The listing builds one solid part. Answer for the finished solid, in the listing's coordinates (mm). Round coordinates to 2 decimals unless told otherwise and drop trailing zeros. Loops run counter-clockwise (first coordinate to the right, second up) from the corner with the lowest first, then second, coordinate; pieces in that order, holes last. Notation, with made-up numbers: M -39.75,-36.5 L -27.75,-36.5 A13 cw -27.75,-20.5 Z; hole C 66.25,19 d11. An arc over 180 degrees is marked long. Put each result on its own line as item: value. Start each with the question number.
(1) Section D-D, the plane x = 19 is taken. Determine the outline of the cut face in (y, z).
(2) Straight lines are drawn through the part: line 1 (Y direction, x = -3, z = 1.35); line 2 (Y direction, x = 0.5, z = 2); line 3 (X direction, y = 76, z = 2.4). For each, find the intervals that lie inside material, in ascending order.
(3) A flat-ended cylindrical pin translates along its axis: P1, Ø13, axis at x = 0, y = -78.93, coming from the -Z side. Find the tip coordinate at first contact, or state that the pin passes through.
(4) Section C-C, the plane y = 71.93 is taken. Determine the outline of the cut face in (x, z).
(5) Section B-B, the plane y = -78.93 is taken. Determine the outline of the cut face in (x, z).
(6) Section A-A, the plane z = 2.25 is taken. Determine the outline of the cut face in (x, y), then the cut area to 3 significant figures.
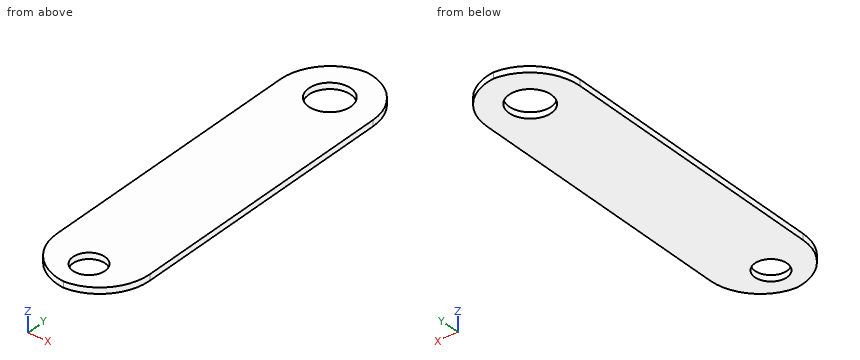
```python
from build123d import *

# Parameters (mm, degrees)
SKETCH1_W           = 46.3
SKETCH1_H           = 189.86
SKETCH1_R           = 10.5
SKETCH1_R_2         = 8
BOSS_EXTRUDE1_DEPTH = 3
FILLET1_R           = 25


with BuildPart() as part:
    # Sketch1 → Boss-Extrude1 (new body)
    with BuildSketch(Plane.XY):
        Rectangle(SKETCH1_W, SKETCH1_H)
        with Locations((0, 71.93)):
            Circle(SKETCH1_R, mode=Mode.SUBTRACT)
        with Locations((0, -78.93)):
            Circle(SKETCH1_R_2, mode=Mode.SUBTRACT)
    extrude(amount=BOSS_EXTRUDE1_DEPTH)

    # Fillet1
    # the kernel refuses this fillet: 25 mm, written as the material it takes off along each edge
    with BuildSketch(Plane(origin=(23.15, -94.93, -62.5), x_dir=(-1, 0, 0), z_dir=(0, 0, 1))) as fillet1_piece_1:
        with BuildLine():
            CenterArc((FILLET1_R, -FILLET1_R), FILLET1_R, 90, 90)
            Line((0, -FILLET1_R), (0, 0))
            Line((0, 0), (FILLET1_R, 0))
        make_face()
    extrude(amount=128, mode=Mode.SUBTRACT)
    with BuildSketch(Plane(origin=(-23.15, -94.93, -62.5), x_dir=(1, 0, 0), z_dir=(0, 0, 1)), Plane(origin=(-23.15, 94.93, -62.5), x_dir=(0, -1, 0), z_dir=(0, 0, 1)), Plane(origin=(23.15, 94.93, -62.5), x_dir=(-1, 0, 0), z_dir=(0, 0, 1))) as fillet1_piece_2:
        with BuildLine():
            CenterArc((FILLET1_R, FILLET1_R), FILLET1_R, 180, 90)
            Line((0, FILLET1_R), (0, 0))
            Line((0, 0), (FILLET1_R, 0))
        make_face()
    extrude(amount=128, mode=Mode.SUBTRACT)


solid = part.part
```
Recorded:
1. outline: M -83.72,0 L 83.72,0 L 83.72,3 L -83.72,3 Z
2. line 1: y = -94.46 to -86.35, -71.51 to 61.87, 81.99 to 94.46
2. line 2: y = -94.82 to -86.91, -70.95 to 61.44, 82.42 to 94.82
2. line 3: x = -22.4 to -9.68, 9.68 to 22.4
3. P1: passes through
4. outline: M -23.07,0 L -10.5,0 L -10.5,3 L -23.07,3 Z; M 10.5,0 L 23.07,0 L 23.07,3 L 10.5,3 Z
5. outline: M -21.47,0 L -8,0 L -8,3 L -21.47,3 Z; M 8,0 L 21.47,0 L 21.47,3 L 8,3 Z
6. outline: M -23.15,-69.93 A25 ccw 0,-94.86 A25 ccw 23.15,-69.93 L 23.15,69.93 A25 ccw 0,94.86 A25 ccw -23.15,69.93 Z; hole C 0,71.93 d21; hole C 0,-78.93 d16
6. area: 7,710 mm²
